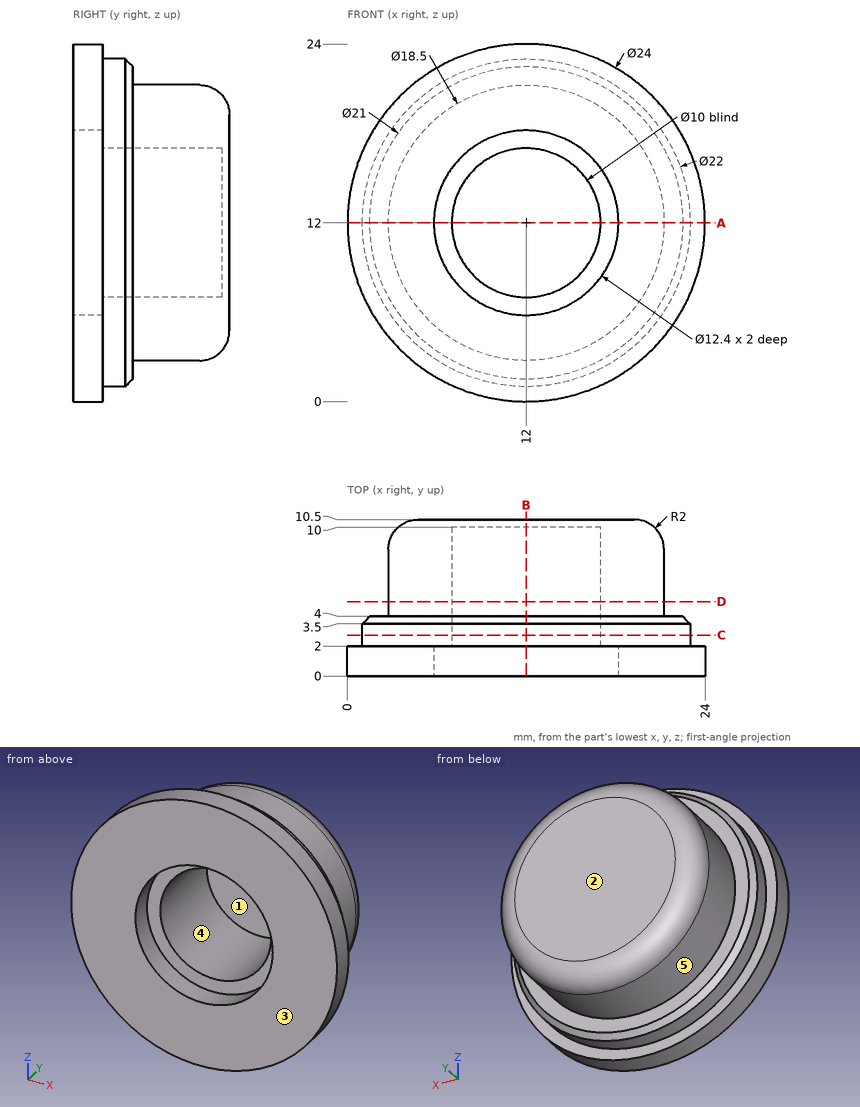
Here's the drawing with two shaded views (mm, measured from the low corner). I have some questions. A direction names the side the tool comes from. Coordinates: 2 decimals unless noted, no trailing zeros. Loops run counter-clockwise (first coordinate to the right, second up) from the corner with the lowest first, then second, coordinate; pieces in that order, holes last. Notation, with made-up numbers: M -6.5,-21 L 1.5,-21 A27 cw 1.5,6 Z; hole C 75.5,-39.5 d8. An arc over 180 degrees is marked long. Return JSON: item names as keys, results as strings. Group by question number.
Item 1: Imagine slicing it at C-C (y = 2.75). Please give me the cut outline in (x, z), and give its area (3 significant figures).
Item 2: Thinking about a two-plate mould opening in X: for the marked faces 3, 4 and 5, which applies, released by +X, released by -X, zero draft, split by the parting line, or undercut?
Item 3: I'm going to push flat-ended pins straight in: pin 1 Ø1 at (x, y) = (11.5, 6) entering from -Z; pin 2 Ø10 at (x, z) = (18.5, 4) entering from -Y; pin 3 Ø5 at (x, y) = (19.5, 6) entering from -Z; pin 4 Ø5 at (x, y) = (19, 7) entering from +Z. Where does each tip first touch, or does it pass through?
Item 4: Imagine slicing it at B-B (x = 12). Please give me the cut outline in (y, z).
Item 5: Imagine slicing it at D-D (y = 5). Please give me the cut outline in (x, z), and give its area (3 significant figures).
Item 6: On a 3-axis mill with a long thin cutter (end or side, diameter ignored), from which of +Z, -Z, +X, -X, +Y, -Y can I reach the whole of each face in a straight line? I mean the marked faces 1 and 2. Say none if no direction works.
Item 7: Imagine slicing it at A-A (z = 12). Please give me the cut outline in (x, y).
Item 8: If I drill on L1, parallel to Z at x = 12, y = 6.75; L2, parallel to Y at x = 11, z = 12; L3, parallel to X at y = 5.5, z = 8, over which ranges is the centre line in solid material (lowest first)? Write a range as from..to.
Verdict:
{
 "1": {"outline": "C 12,12 d22; hole C 12,12 d10", "area": "302 mm^2"},
 "2": {"face 3": "zero draft", "face 4": "undercut", "face 5": "split by the parting line"},
 "3": {"pin 1": "stops at z = 2.75", "pin 2": "stops at y = 0", "pin 3": "stops at z = 3.36", "pin 4": "stops at z = 20.08"},
 "4": {"outline": "M 0,0 L 2,0 L 2,1 L 3.5,1 L 4,1.5 L 4,2.75 L 8.5,2.75 A2 ccw 10.5,4.75 L 10.5,19.25 A2 ccw 8.5,21.25 L 4,21.25 L 4,22.5 L 3.5,23 L 2,23 L 2,24 L 0,24 L 0,18.2 L 2,18.2 L 2,17 L 10,17 L 10,7 L 2,7 L 2,5.8 L 0,5.8 Z"},
 "5": {"outline": "C 12,12 d18.5; hole C 12,12 d10", "area": "190 mm^2"},
 "6": {"face 1": "-Y", "face 2": "+Z, -Z, +X, -X, +Y"},
 "7": {"outline": "M 0,0 L 5.8,0 L 5.8,2 L 7,2 L 7,10 L 17,10 L 17,2 L 18.2,2 L 18.2,0 L 24,0 L 24,2 L 23,2 L 23,3.5 L 22.5,4 L 21.25,4 L 21.25,8.5 A2 ccw 19.25,10.5 L 4.75,10.5 A2 ccw 2.75,8.5 L 2.75,4 L 1.5,4 L 1,3.5 L 1,2 L 0,2 Z"},
 "8": {"L1": "z = 2.75..7, 17..21.25", "L2": "y = 10..10.5", "L3": "x = 3.66..9, 15..20.34"}
}
